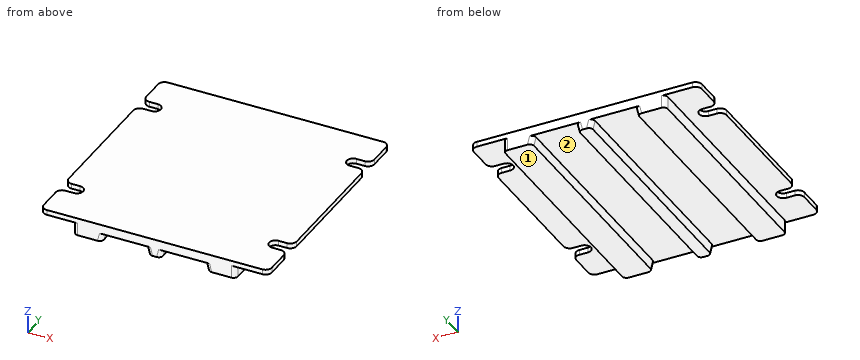
```python
from build123d import *

# Parameters (mm, degrees)
F1_DEPTH = 56
F3_DEPTH = 25
F4_R     = 1.5
F5_R     = 1


with BuildPart() as f1:
    # F0 (on Front) → F1 (new body)
    with BuildSketch(Plane.XZ):
        Polygon((-1.5, 0), (0, 0), (0, 4.2), (-27, 4.2), (-27, 3), (-19.2, 3), (-19.2, 0), (-12.5, 0), (-12, 2), (-2, 2), align=None)
        Polygon((0, 4.2), (0, 0), (1.5, 0), (2, 2), (12, 2), (12.5, 0), (19.2, 0), (19.2, 3), (27, 3), (27, 4.2), align=None)
    extrude(amount=F1_DEPTH)

    # F2 (on face) → F3 (cut)
    with BuildSketch(Plane.XY.offset(4.2)):
        with BuildLine():
            Line((27, -47.5), (27, -44.5))
            Line((27, -44.5), (23.5, -44.5))
            ThreePointArc((23.5, -44.5), (22.4393398282, -44.9393398282), (22, -46))
            ThreePointArc((22, -46), (22.4393398282, -47.0606601718), (23.5, -47.5))
            Line((23.5, -47.5), (27, -47.5))
        make_face()
        with BuildLine():
            Line((27, -11.5), (27, -8.5))
            Line((27, -8.5), (23.5, -8.5))
            ThreePointArc((23.5, -8.5), (22.4393398282, -8.9393398282), (22, -10))
            ThreePointArc((22, -10), (22.4393398282, -11.0606601718), (23.5, -11.5))
            Line((23.5, -11.5), (27, -11.5))
        make_face()
        with BuildLine():
            ThreePointArc((-22, -10), (-22.4393398282, -8.9393398282), (-23.5, -8.5))
            Line((-23.5, -8.5), (-27, -8.5))
            Line((-27, -8.5), (-27, -11.5))
            Line((-27, -11.5), (-23.5, -11.5))
            ThreePointArc((-23.5, -11.5), (-22.4393398282, -11.0606601718), (-22, -10))
        make_face()
        with BuildLine():
            Line((-23.5, -44.5), (-27, -44.5))
            Line((-27, -44.5), (-27, -47.5))
            Line((-27, -47.5), (-23.5, -47.5))
            ThreePointArc((-23.5, -47.5), (-22.4393398282, -47.0606601718), (-22, -46))
            ThreePointArc((-22, -46), (-22.4393398282, -44.9393398282), (-23.5, -44.5))
        make_face()
    extrude(amount=-F3_DEPTH, mode=Mode.SUBTRACT)

    # F4
    f4_edges = [f1.edges().sort_by_distance(p)[0] for p in [
        (-27, -47.5, 3.6),
        (-27, -44.5, 3.6),
        (27, -47.5, 3.6),
        (27, -44.5, 3.6),
        (27, -11.5, 3.6),
        (27, -8.5, 3.6),
        (-27, -11.5, 3.6),
        (-27, -8.5, 3.6),
        (27, -56, 3.6),
        (-27, -56, 3.6),
        (-27, 0, 3.6),
        (27, 0, 3.6),
    ]]
    fillet(f4_edges, radius=F4_R)

    # F5
    f5_edges = [f1.edges().sort_by_distance(p)[0] for p in [
        (12.25, 0, 1),
        (19.2, 0, 1.5),
        (1.75, 0, 1),
        (-1.75, 0, 1),
        (-12.25, 0, 1),
        (-19.2, 0, 1.5),
        (-19.2, -56, 1.5),
        (-12.25, -56, 1),
        (-1.75, -56, 1),
        (1.75, -56, 1),
        (12.25, -56, 1),
        (19.2, -56, 1.5),
    ]]
    fillet(f5_edges, radius=F5_R)


solid = f1.part
```
Could you check a few things on this model? Use its own coordinates, in mm. Face numbers are marked on the shaded views. Round coordinates to 2 decimals unless told otherwise and drop trailing zeros. Order: outer loops, then holes, each group sorted by start corner. A loop starts at its lowest first (then second) coordinate and runs counter-clockwise, first axis right, second up. Notation, with made-up numbers: M 55.5,15 L 86.5,15 A27 cw 86.5,45 Z; hole C -33,-11.5 d1. An arc over 180 degrees is marked long. One line per question, with ' | ' between items. Start each with the question number.
(1) Please list where these lines run through material, in increasing order: line 1 along X through (y, z) = (-43, 0.8); line 2 along X through (y, z) = (-52, 0.45); line 3 along Z through (x, y) = (-3.5, -52.5).
(2) Suppose I cut it at A-A on y = -32.5. List the corners of the cut face in (x, z) for me, then the cut area to 3 significant figures.
(3) Suppose I cut it at B-B on x = 10. List the corners of the cut face in (y, z) for me.
(4) For P1, Ø9.5, axis at x = -9.5, y = -25.5, coming from the -Z side; P2, Ø0.9, axis at y = -17.5, z = 1.5, coming from the +X side, each with a flat end and sliding along its axis, tell me the tip position at first contact or that it passes through.
(5) Suppose I cut it at C-C on z = 1.1. Count the separate pieces of the cut face and the enclosed holes in it, then the cut area to 3 significant figures.
(6) Thinking about a two-plate mould opening in X: for the marked faces 1 and 2, which applies, +X half, -X half, draft (parallel to the pull), parting line (faces both ways), or undercut?
Geometry results:
1) line 1: -19.2 to -12.3, -1.7 to 1.7, 12.3 to 19.2 | line 2: -19.2 to -12.39, -1.61 to 1.61, 12.39 to 19.2 | line 3: 2 to 4.2
2) outline: M -27,3 L -19.2,3 L -19.2,0 L -12.5,0 L -12,2 L -2,2 L -1.5,0 L 1.5,0 L 2,2 L 12,2 L 12.5,0 L 19.2,0 L 19.2,3 L 27,3 L 27,4.2 L -27,4.2 Z | area: 138 mm²
3) outline: M -56,2 L 0,2 L 0,4.2 L -56,4.2 Z
4) P1: z = 0 | P2: x = 19.2
5) separate pieces: 3 | enclosed holes: 0 | area: 977 mm²
6) face 1: draft | face 2: undercut
